Here's the drawing with two shaded views (mm, measured from the low corner). I have some questions. A direction names the side the tool comes from. Round coordinates to 2 decimals unless told otherwise and drop trailing zeros. Write each loop counter-clockwise with the first axis right and the second up, starting at its lowest first coordinate (ties: lowest second). Pieces come first, ordered by that corner, then holes. Notation, with made-up numbers: M -7,81.25 L 43,81.25 A23 cw 43,89.25 Z; hole C 57.5,-6 d1. An arc over 180 degrees is marked long. Write item = value, one per line. Start each with the question number.
(1) I want a section at D-D (z = 22). List the corners of the cut face in (x, y) for me, and give its area (3 significant figures).
(2) If we mould it in two halves opening along X, with no side actions, what happens to the marked faces 1, 2, 3 and 4? For each: released by +X, released by -X, zero draft, split by the parting line, or undercut.
(3) I want a section at C-C (z = 8.25). List the corners of the cut face in (x, y) for me, and give its area (3 significant figures).
(4) I want a section at B-B (z = 12.5). List the corners of the cut face in (x, y) for me.
(5) I need wall thicknesses on line 1 along X through (y, z) = (1.2, 12.5); line 2 along Z through (x, y) = (5, 1); line 3 along X through (y, z) = (2.4, 11.5). Which ranges of each line are inside material? Lowest first, please.
(6) On a 3-axis mill with a long thin cutter (end or side, diameter ignored), from which of +Z, -Z, +X, -X, +Y, -Y can I reach the whole of each face in a straight line? I mean the marked faces 5 and 6. Say none if no direction works.
(7) Will these pins go through, and if not, where does the flat tip stop? pin 1 Ø6 at (x, z) = (20, 13) entering from +Y; pin 2 Ø1.5 at (y, z) = (1, 22.5) entering from +X.
(8) I want a section at A-A (y = 1.2). List the corners of the cut face in (x, z) for me, and give its area (3 significant figures).
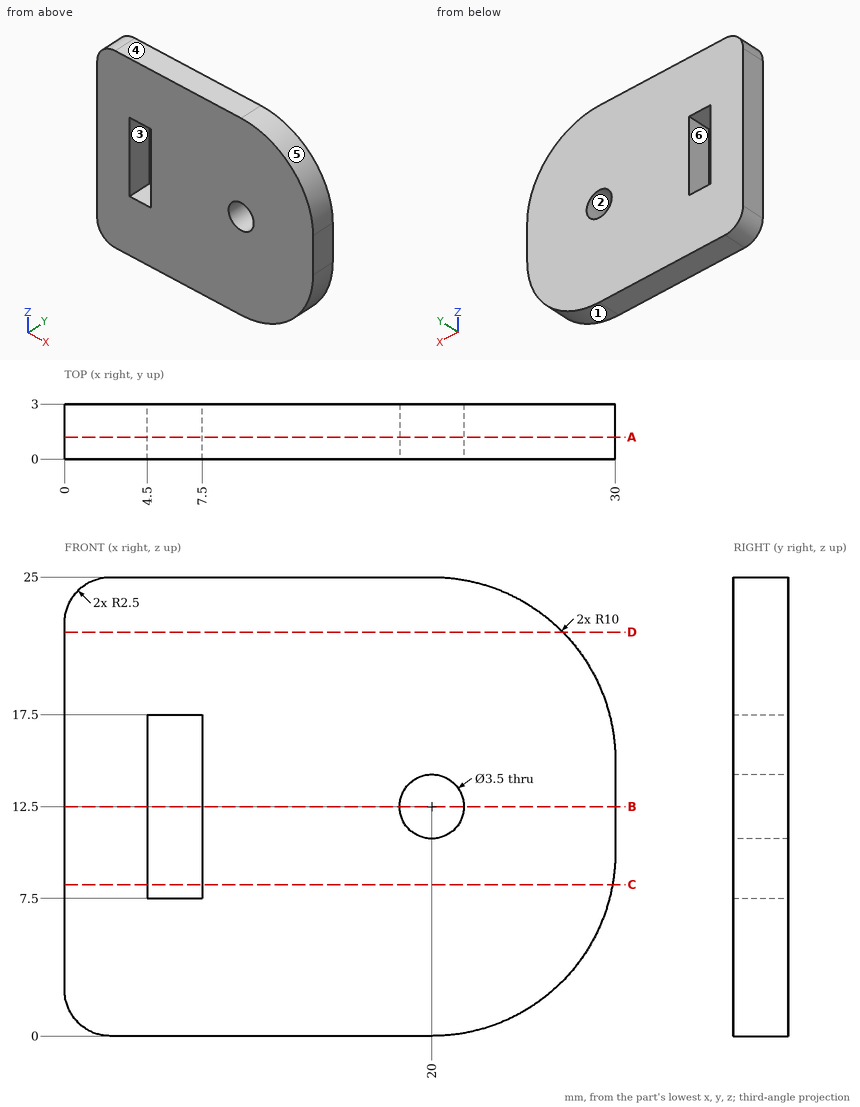
Returned:
q1.outline = M 0,0 L 27.14,0 L 27.14,3 L 0,3 Z
q1.area = 81.4 mm²
q2.face_1 = released by +X
q2.face_2 = undercut
q2.face_3 = undercut
q2.face_4 = zero draft
q3.outline = M 0,0 L 4.5,0 L 4.5,3 L 0,3 Z; M 7.5,0 L 29.85,0 L 29.85,3 L 7.5,3 Z
q3.area = 80.5 mm²
q4.outline = M 0,0 L 4.5,0 L 4.5,3 L 0,3 Z; M 7.5,0 L 18.25,0 L 18.25,3 L 7.5,3 Z; M 21.75,0 L 30,0 L 30,3 L 21.75,3 Z
q5.line_1 = 0 to 4.5, 7.5 to 18.25, 21.75 to 30
q5.line_2 = 0 to 7.5, 17.5 to 25
q5.line_3 = 0 to 4.5, 7.5 to 18.56, 21.44 to 30
q6.face_5 = +Z, +X, +Y, -Y
q6.face_6 = +Y, -Y
q7.pin_1 = 3
q7.pin_2 = 27.38
q8.outline = M 0,2.5 A2.5 ccw 2.5,0 L 20,0 A10 ccw 30,10 L 30,15 A10 ccw 20,25 L 2.5,25 A2.5 ccw 0,22.5 Z; hole M 4.5,7.5 L 7.5,7.5 L 7.5,17.5 L 4.5,17.5 Z; hole C 20,12.5 d3.5
q8.area = 665 mm²
